Can you work these out from the model? Positions are in its coordinate system, mm. Face numbers are marked on the shaded views. Round coordinates to 2 decimals unless told otherwise and drop trailing zeros. Loops run counter-clockwise (first coordinate to the right, second up) from the corner with the lowest first, then second, coordinate; pieces in that order, holes last. Notation, with made-up numbers: (60.25, 75.25) -> (95.25, 75.25) arc R18 cw to (95.25, 87.25) -> close; hole circle Ø4 at (18.25, 44.25). An arc over 180 degrees is marked (long way). Write item = value, one per line.
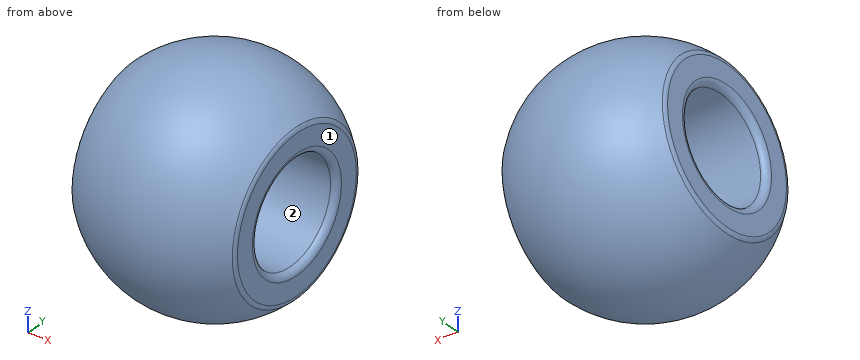
Autodesk Inventor part; units mm, degrees
ref_plane "ball_XY" through (0, 0, 0) normal (1, 0, 0) x (0, 0, -1)
ref_plane "ball_YZ" through (0, 0, 0) normal (0, 0, -1) x (0, 1, 0)
ref_plane "ball_ZX" through (0, 0, 0) normal (0, 1, 0) x (1, 0, 0)
sketch "Sketch_1" plane through (0, 0, 0) normal (0, 0, 1) x (1, 0, 0)
  line L0 (4, 0) -> (-4, 0)
  arc A0 (-4, 2.8) -> (-3.7, 2.5) centre (-3.7, 2.8) ccw
  line L1 (-3.7, 2.5) -> (3.7, 2.5)
  arc A1 (3.7, 2.5) -> (4, 2.8) centre (3.7, 2.8) ccw
  line L2 (4, 2.8) -> (4, 3.733)
  arc A2 (4, 3.733) -> (3.9112, 3.9461) centre (3.7, 3.733) ccw
  arc A3 (3.9112, 3.9461) -> (-3.9112, 3.9461) centre (0, 0) ccw
  arc A4 (-3.9112, 3.9461) -> (-4, 3.733) centre (-3.7, 3.733) ccw
  line L3 (-4, 3.733) -> (-4, 2.8)
revolve "Revolution1" add sketch "Sketch_1" angle 360 about axis through (4, 0, 0) along (1, 0, 0)
ref_plane "ball_XY" through (0, 0, 0) normal (1, 0, 0) x (0, 0, -1)
ref_plane "ball_YZ" through (0, 0, 0) normal (0, 0, -1) x (0, 1, 0)
ref_plane "ball_ZX" through (0, 0, 0) normal (0, 1, 0) x (1, 0, 0)
properties part number "RBPB5ball"
1. We'd pull the mould along Z, two halves only. Please class the marked faces 1 and 2: released by +Z, released by -Z, zero draft, split by the parting line, or undercut.
Entries:
face_1 = zero draft
face_2 = undercut
2. I'm going to push flat-ended pins straight in: pin 1 (2 mm diameter, centred on x = 1, y = -3.5, fed in from -Z); pin 2 (1 mm diameter, centred on x = -1.5, z = -2.5, fed in from -Y); pin 3 (2 mm diameter, centred on x = 2, y = 0, fed in from +Z). Where does each tip first touch, or does it pass through?
Entries:
pin_1 = -4.89
pin_2 = -5
pin_3 = 5.47
3. Suppose I cut it at A-A, the plane z = 0. List the corners of the cut face in (x, y) for me.
Entries:
outline = (-4, -3.73) arc R0.3 ccw to (-3.91, -3.95) arc R5.56 ccw to (3.91, -3.95) arc R0.3 ccw to (4, -3.73) -> (4, -2.8) arc R0.3 ccw to (3.7, -2.5) -> (-3.7, -2.5) arc R0.3 ccw to (-4, -2.8) -> close; (-4, 2.8) arc R0.3 ccw to (-3.7, 2.5) -> (3.7, 2.5) arc R0.3 ccw to (4, 2.8) -> (4, 3.73) arc R0.3 ccw to (3.91, 3.95) arc R5.56 ccw to (-3.91, 3.95) arc R0.3 ccw to (-4, 3.73) -> close
4. Suppose I cut it at D-D, the plane y = -4.25. List the corners of the cut face in (x, z) for me, and give its area (3 significant figures).
Entries:
outline = circle Ø7.16 at (0, 0)
area = 40.2 mm²
5. Suppose I cut it at C-C, the plane x = 1. List the corners of the cut face in (y, z) for me.
Entries:
outline = circle Ø10.93 at (0, 0); hole circle Ø5 at (0, 0)
6. I need wall thicknesses on line 1 (Z direction, x = -2.5, y = -1.5); line 2 (Z direction, x = -2, y = -1.5); line 3 (X direction, y = -2.5, z = -3). Which ranges of each line are inside material? Lowest first, please. Write a range as [from, to].
Entries:
line_1 = [-4.73, -2], [2, 4.73]
line_2 = [-4.96, -2], [2, 4.96]
line_3 = [-3.95, 3.95]
